from build123d import *

# Parameters (mm, degrees)
F0_R         = 2.5
F1_DEPTH     = 35
F3_DEPTH     = 25
F4_T4_DEPTH  = 88.824838337
F4_T9_DEPTH  = 88.824838337
F4_T12_ANGLE = 170.716427301
F5_R         = 15
F6_DEPTH     = 20


# Not quite as in the source:
# - a fillet or chamfer that OpenCascade refuses, or shapes differently, is made with other operations: its cross-section is extruded or revolved along the edge and cut away or added


with BuildPart() as f1:
    # F0 (on Top) → F1 (new body)
    with BuildSketch(Plane.XY):
        with BuildLine():
            Line((0.6698729811, 11.1602540378), (-75.4046293156, 4.9836006177))
            ThreePointArc((-75.4046293156, 4.9836006177), (-80, 0), (-75.4046293156, -4.9836006177))
            Line((-75.4046293156, -4.9836006177), (0.6698729811, -11.1602540378))
            Line((0.6698729811, -11.1602540378), (10.6698729811, -28.4807621135))
            Line((10.6698729811, -28.4807621135), (15, -25.9807621135))
            Line((15, -25.9807621135), (0, 0))
            Line((0, 0), (15, 25.9807621135))
            Line((15, 25.9807621135), (10.6698729811, 28.4807621135))
            Line((10.6698729811, 28.4807621135), (0.6698729811, 11.1602540378))
        make_face()
        with Locations((-75, 0)):
            Circle(F0_R, mode=Mode.SUBTRACT)
    extrude(amount=F1_DEPTH)

    # F2 (on face) → F3 (join)
    with BuildSketch(Plane.XY.offset(35)):
        Polygon((15, -25.9807621135), (0, 0), (15, 25.9807621135), (10.6698729811, 28.4807621135), (0.6698729811, 11.1602540378), (-5.7735026919, 0), (0.6698729811, -11.1602540378), (10.6698729811, -28.4807621135), align=None)
    extrude(amount=F3_DEPTH)

    # F4: fillet of radius 5 on 2 edges, made by hand


with BuildPart() as f4_tool2:
    # F4_s3 → F4_t4 (new body)
    with BuildSketch(Plane(origin=(-74.5088253508, 6.0495327217, 0), x_dir=(0, 0, 1), z_dir=(0.9967201235, -0.0809258631, 0))):
        with BuildLine():
            ThreePointArc((35, 6.0694397342), (33.5355339059, 9.6049736401), (30, 11.0694397342))
            Line((30, 11.0694397342), (35, 11.0694397342))
            Line((35, 11.0694397342), (35, 6.0694397342))
        make_face()
    extrude(amount=F4_T4_DEPTH)

    split(bisect_by=Plane(origin=(-4.3301270189, -2.5, 0), x_dir=(0, 0, 1), z_dir=(-0.8660254038, -0.5, 0)), keep=Keep.TOP)


with BuildPart() as f1_1:
    add(f1.part)

    # F4_t1: cut F4_tool2
    add(f4_tool2.part, mode=Mode.SUBTRACT)


with BuildPart() as f4_tool7:
    # F4_s8 → F4_t9 (new body)
    with BuildSketch(Plane(origin=(14.0246784902, 1.1386939874, 0), x_dir=(0, 0, 1), z_dir=(-0.9967201235, -0.0809258631, 0))):
        with BuildLine():
            ThreePointArc((30, 11.0694397342), (33.5355339059, 9.6049736401), (35, 6.0694397342))
            Line((35, 6.0694397342), (35, 11.0694397342))
            Line((35, 11.0694397342), (30, 11.0694397342))
        make_face()
    extrude(amount=F4_T9_DEPTH)

    split(bisect_by=Plane(origin=(-4.3301270189, 2.5, 0), x_dir=(0, 0, 1), z_dir=(-0.8660254038, 0.5, 0)), keep=Keep.TOP)


with BuildPart() as f1_2:
    add(f1_1.part)

    # F4_t6: cut F4_tool7
    add(f4_tool7.part, mode=Mode.SUBTRACT)

    # F4_s11 → F4_t12 (revolve, cut)
    with BuildSketch(Plane(origin=(-74.5088253508, -6.0495327217, 0), x_dir=(0, 0, 1), z_dir=(0.9967201235, 0.0809258631, 0))):
        with BuildLine():
            ThreePointArc((35, -6.0694397342), (33.5355339059, -9.6049736401), (30, -11.0694397342))
            Line((30, -11.0694397342), (35, -11.0694397342))
            Line((35, -11.0694397342), (35, -6.0694397342))
        make_face()
    revolve(axis=Axis((-75, 0, 35), (0, 0, 1)), revolution_arc=F4_T12_ANGLE, mode=Mode.SUBTRACT)

    # F5 (on Top) → F6 (cut)
    with BuildSketch(Plane.XY):
        with Locations((6, 0)):
            Circle(F5_R)
    extrude(amount=F6_DEPTH, mode=Mode.SUBTRACT)


solid = f1_2.part
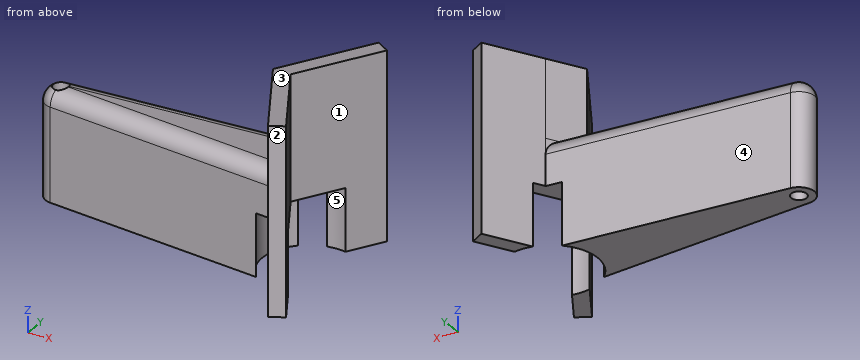
The model under review builds one solid part; all positions refer to its coordinate system, in mm. Face numbers are marked on the shaded views. A direction names the side the tool comes from. Give positions to 0.01 mm unless a question says otherwise; leave off trailing zeros. Order: outer loops, then holes, each group sorted by start corner. A loop starts at its lowest first (then second) coordinate and runs counter-clockwise, first axis right, second up. Notation, with made-up numbers: M 55,19.25 L 100,19.25 A19 cw 100,47.25 Z; hole C 39.5,67.25 d3. An arc over 180 degrees is marked long. One line per question, with ' | ' between items. Start each with the question number.
1) For the marked faces 4 and 5, list the 3-axis set-ups (+Z, -Z, +X, -X, +Y, -Y) from which the entire face can be reached by the end or side of a thin tool; tool diameter is ignored.
2) Mouldability with a two-part tool opening along Y and no side actions: class the marked faces 1, 2 and 3 as pulls with the +Y half, pulls with the -Y half, needs draft (parallel to the pull), parting line crosses it, or undercut.
3) Wall thickness on L1, parallel to Y at x = -75, z = 14; L2, parallel to Z at x = -6, y = 2.5; L3, parallel to Z at x = 3.5, y = -7.5: over which ranges is each line inside the solid? List them lowest first. Write a range as from..to.
4) Consider section A-A, the plane z = 45.5. Give the boundary of the cut face in (x, y), then the cut area to 3 significant figures.
5) Consider section B-B, the plane y = 18. Give the boundary of the cut face in (x, z), then the cut area to 3 significant figures.
6) Clearance check with flat-ended pins moving along their axes: P1, Ø1.5, axis at x = -49, z = 36.5, coming from the +Y side; P2, Ø5, axis at x = -12.5, z = 14, coming from the -Y side; P3, Ø8, axis at x = -6.5, z = 6.5, coming from the +Y side; P4, Ø5.5, axis at x = 1.5, y = 3.5, coming from the -Z side. State where each tip first meets the part, or that it passes through.
Found:
1) face 4: +Z, -Z, -X, +Y | face 5: -Z
2) face 1: undercut | face 2: pulls with the -Y half | face 3: needs draft
3) L1: y = -5.02..-2.5, 2.5..5.02 | L2: z = 20..35 | L3: z = 20..60
4) outline: M -5.77,0 L 10.67,-28.48 L 15,-25.98 L 0,0 L 15,25.98 L 10.67,28.48 Z | area: 314 mm²
5) outline: M 4.62,0 L 10.39,0 L 10.39,60 L 4.62,60 Z | area: 346 mm²
6) P1: passes through | P2: stops at y = -10.29 | P3: stops at y = 10.74 | P4: stops at z = 20
